from build123d import *

# Parameters (mm, degrees)
SKETCH_1_R          = 3.5
SKETCH_1_R_2        = 19
EXTRUDE_1_DEPTH     = 11.5
SKETCH_2_R          = 42.113859259
CUT_EXTRUDE_1_DEPTH = 6
SKETCH_3_R          = 15.5
CUT_EXTRUDE_3_DEPTH = 1
CUT_EXTRUDE_4_DEPTH = 1
FILLET_1_R          = 5
SKETCH_5_R          = 13.5
CUT_EXTRUDE_6_DEPTH = 21


with BuildPart() as part:
    # Эскиз1 → Бобышка-Вытянуть1 (new body)
    # profile 1 of 3: a face of its own
    with BuildSketch(Plane(origin=(0, 0, 0), x_dir=(1, 0, 0), z_dir=(0, 1, 0))):
        with BuildLine():
            ThreePointArc((-29.93902439, 6.351219512), (-31.061737619, 5.649390095), (-31.5, 4.4))
            Line((-31.5, 4.4), (-31.5, -4.4))
            ThreePointArc((-31.5, -4.4), (-31.061737619, -5.649390095), (-29.93902439, -6.351219512))
            Line((-29.93902439, -6.351219512), (-16.529826375, -9.368289066))
            ThreePointArc((-16.529826375, -9.368289066), (-19, 0), (-16.529826375, 9.368289066))
            Line((-16.529826375, 9.368289066), (-29.93902439, 6.351219512))
        make_face()
        with Locations(Location((-24, 0, 0), (0, 0, 270))):
            Circle(SKETCH_1_R, mode=Mode.SUBTRACT)
    # profile 2 of 3: a face of its own
    with BuildSketch(Plane(origin=(0, 0, 0), x_dir=(1, 0, 0), z_dir=(0, 1, 0))):
        Circle(SKETCH_1_R_2)
    # profile 3 of 3: a face of its own
    with BuildSketch(Plane(origin=(0, 0, 0), x_dir=(1, 0, 0), z_dir=(0, 1, 0))):
        with BuildLine():
            Line((29.93902439, 6.351219512), (16.529826375, 9.368289066))
            ThreePointArc((16.529826375, 9.368289066), (18.372080736, 4.844238788), (19, 0))
            ThreePointArc((19, 0), (18.372080736, -4.844238788), (16.529826375, -9.368289066))
            Line((16.529826375, -9.368289066), (29.93902439, -6.351219512))
            ThreePointArc((29.93902439, -6.351219512), (31.061737619, -5.649390095), (31.5, -4.4))
            Line((31.5, -4.4), (31.5, 4.4))
            ThreePointArc((31.5, 4.4), (31.061737619, 5.649390095), (29.93902439, 6.351219512))
        make_face()
        with Locations(Location((24, 0, 0), (0, 0, 270))):
            Circle(SKETCH_1_R, mode=Mode.SUBTRACT)
    extrude(amount=EXTRUDE_1_DEPTH)

    # Эскиз2 → Вырез-Вытянуть1 (cut)
    with BuildSketch(Plane(origin=(0, 11.5, 0), x_dir=(1, 0, 0), z_dir=(0, 1, 0))):
        Circle(SKETCH_2_R)
        with BuildLine():
            ThreePointArc((17.208333333, 3.1817077), (0, 17.5), (-17.208333333, 3.1817077))
            ThreePointArc((-17.208333333, 3.1817077), (-16.5, 0), (-17.208333333, -3.1817077))
            ThreePointArc((-17.208333333, -3.1817077), (0, -17.5), (17.208333333, -3.1817077))
            ThreePointArc((17.208333333, -3.1817077), (16.5, 0), (17.208333333, 3.1817077))
        make_face(mode=Mode.SUBTRACT)
    extrude(amount=-CUT_EXTRUDE_1_DEPTH, mode=Mode.SUBTRACT)

    # Эскиз3 → Вырез-Вытянуть3 (cut)
    with BuildSketch(Plane(origin=(0, 11.5, 0), x_dir=(1, 0, 0), z_dir=(0, 1, 0))):
        with Locations(Location((0, 0, 0), (0, 0, 270))):
            Circle(SKETCH_3_R)
    extrude(amount=-CUT_EXTRUDE_3_DEPTH, mode=Mode.SUBTRACT)

    # Эскиз4 → Вырез-Вытянуть4 (cut)
    with BuildSketch(Plane.XZ):
        with BuildLine():
            Line((-20.848643232, -5.321555273), (-15.718229563, -6.475898348))
            ThreePointArc((-15.718229563, -6.475898348), (-14.636214456, -8.647613914), (-13.256050789, -10.643172341))
            ThreePointArc((-13.256050789, -10.643172341), (-12.584964511, -11.011180012), (-11.850214134, -10.796871074))
            ThreePointArc((-11.850214134, -10.796871074), (-10.750830182, -10.362248437), (-9.598076211, -10.624355653))
            Line((-9.598076211, -10.624355653), (-4.401923789, -13.624355653))
            ThreePointArc((-4.401923789, -13.624355653), (-3.598555295, -14.491616268), (-3.425257564, -15.661022017))
            ThreePointArc((-3.425257564, -15.661022017), (-3.243479361, -16.404488978), (-2.58923223, -16.801662908))
            ThreePointArc((-2.58923223, -16.801662908), (8.351526577, -14.807160559), (15.718229563, -6.475898348))
            Line((15.718229563, -6.475898348), (20.848643232, -5.321555273))
            ThreePointArc((20.848643232, -5.321555273), (21.605203579, -4.563390663), (21.242016303, -3.555773605))
            ThreePointArc((21.242016303, -3.555773605), (19.5, 0), (21.242016303, 3.555773605))
            ThreePointArc((21.242016303, 3.555773605), (21.605203579, 4.563390663), (20.848643232, 5.321555273))
            Line((20.848643232, 5.321555273), (15.718229563, 6.475898348))
            ThreePointArc((15.718229563, 6.475898348), (14.636214456, 8.647613914), (13.256050789, 10.643172341))
            ThreePointArc((13.256050789, 10.643172341), (12.584964511, 11.011180012), (11.850214134, 10.796871074))
            ThreePointArc((11.850214134, 10.796871074), (10.750830182, 10.362248437), (9.598076211, 10.624355653))
            Line((9.598076211, 10.624355653), (4.401923789, 13.624355653))
            ThreePointArc((4.401923789, 13.624355653), (3.598555295, 14.491616268), (3.425257564, 15.661022017))
            ThreePointArc((3.425257564, 15.661022017), (3.243479361, 16.404488978), (2.58923223, 16.801662908))
            ThreePointArc((2.58923223, 16.801662908), (-8.351526577, 14.807160559), (-15.718229563, 6.475898348))
            Line((-15.718229563, 6.475898348), (-20.848643232, 5.321555273))
            ThreePointArc((-20.848643232, 5.321555273), (-21.605203579, 4.563390663), (-21.242016303, 3.555773605))
            ThreePointArc((-21.242016303, 3.555773605), (-19.5, 0), (-21.242016303, -3.555773605))
            ThreePointArc((-21.242016303, -3.555773605), (-21.605203579, -4.563390663), (-20.848643232, -5.321555273))
        make_face()
        with BuildLine():
            Line((6.035898385, 18.454482672), (12.964101615, 14.454482672))
            Line((12.964101615, 14.454482672), (11.464101615, 11.856406461))
            ThreePointArc((11.464101615, 11.856406461), (10.856895256, 11.390480634), (10.098076211, 11.490381057))
            Line((10.098076211, 11.490381057), (4.901923789, 14.490381057))
            ThreePointArc((4.901923789, 14.490381057), (4.435997962, 15.097587415), (4.535898385, 15.856406461))
            Line((4.535898385, 15.856406461), (6.035898385, 18.454482672))
        make_face()
        with BuildLine():
            Line((-6.035898385, -18.454482672), (-4.535898385, -15.856406461))
            ThreePointArc((-4.535898385, -15.856406461), (-4.435997962, -15.097587415), (-4.901923789, -14.490381057))
            Line((-4.901923789, -14.490381057), (-10.098076211, -11.490381057))
            ThreePointArc((-10.098076211, -11.490381057), (-10.856895256, -11.390480634), (-11.464101615, -11.856406461))
            Line((-11.464101615, -11.856406461), (-12.964101615, -14.454482672))
            Line((-12.964101615, -14.454482672), (-6.035898385, -18.454482672))
        make_face()
    extrude(amount=-CUT_EXTRUDE_4_DEPTH, mode=Mode.SUBTRACT)

    # Скругление1
    fillet_1_edges = [part.edges().sort_by_distance(p)[0] for p in [
        (-16.529826375, 2.75, -9.368289066),
        (16.529826375, 2.75, -9.368289066),
        (16.529826375, 2.75, 9.368289066),
        (-16.529826375, 2.75, 9.368289066),
    ]]
    fillet(fillet_1_edges, radius=FILLET_1_R)

    # Эскиз5 → Вырез-Вытянуть6 (cut)
    with BuildSketch(Plane(origin=(0, 10.5, 0), x_dir=(1, 0, 0), z_dir=(0, 1, 0))):
        with Locations(Location((0, 0, 0), (0, 0, 270))):
            Circle(SKETCH_5_R)
    extrude(amount=-CUT_EXTRUDE_6_DEPTH, mode=Mode.SUBTRACT)


solid = part.part
Work out the finished part from the listing and answer in its coordinate system (mm). A direction names the side the tool comes from. Round coordinates to 2 decimals unless told otherwise and drop trailing zeros. Write each loop counter-clockwise with the first axis right and the second up, starting at its lowest first coordinate (ties: lowest second). Pieces come first, ordered by that corner, then holes.
1) Given pin 1 Ø3 at (y, z) = (7.5, 13.5) entering from +X; pin 2 Ø6 at (y, z) = (10, -12) entering from +X; pin 3 Ø5 at (x, z) = (17.5, 13) entering from +Y; pin 4 Ø5.5 at (x, z) = (8, 16) entering from -Y, each flat-ended and moving along its own axis, determine where each tip first touches the part or whether it passes through.
2) A cutting plane is placed at C-C (z = 12.5). Give the vertices of the cut face in (x, y).
3) A cutting plane is placed at D-D (x = -25). Give the vertices of the cut face in (y, z), plus the area to 3 significant figures.
4) A cutting plane is placed at A-A (x = 0). Give the vertices of the cut face in (y, z).
5) Straight lines are drawn through the part: line 1 (X direction, y = 3.3, z = 0); line 2 (X direction, y = 1.25, z = -1); line 3 (X direction, y = 6.5, z = 0). For each, find the intervals that lie inside material, in ascending order.
6) The mould has two halves that part along Z. Classify faces 5 (the cylindrical face through (-19.5, 0.5, 0.1)), 6 (the cylindrical face through (0.34, 8.542, -17.497)), 7 (the flat face through (-24.321, 2.712, 7.615)): pulls with the +Z half, pulls with the -Z half, needs draft (parallel to the pull), parting line crosses it, or undercut.
7) A tool of negligible diameter and unlimited length cuts with its end or side. For faces 1 (the flat face through (-18.248, 0.493, 5.907)), 2 (the flat face through (13, 10.5, -5)), 3 (the flat face through (5.17, 0.493, 16.955)), 4 (the cylindrical face through (-16.5, 8.5, 0)), from which of +Z, -Z, +X, -X, +Y, -Y can it reach the whole face along a straight path? Write none if from no direction.
8) A cutting plane is placed at B-B (y = 2.5). Give the vertices of the cut face in (x, z), plus the area to 3 significant figures.
Completed:
1. pin 1: stops at x = 12.74
1. pin 2: stops at x = 15.01
1. pin 3: passes through
1. pin 4: stops at y = 1
2. outline: (-14.31, 0) - (-11.52, 0) - (-11.52, 1) - (-5.1, 1) - (-5.1, 10.5) - (-9.17, 10.5) - (-9.17, 11.5) - (-12.25, 11.5) - (-12.25, 5.5) - (-14.31, 5.5) - close; (5.1, 1) - (6.35, 1) - (6.35, 0) - (8.35, 0) - (8.35, 1) - (11.84, 1) - (11.84, 0) - (14.31, 0) - (14.31, 5.5) - (12.25, 5.5) - (12.25, 11.5) - (9.17, 11.5) - (9.17, 10.5) - (5.1, 10.5) - close
3. outline: (0, -7.46) - (5.5, -7.46) - (5.5, -3.35) - (0, -3.35) - close; (0, 3.35) - (5.5, 3.35) - (5.5, 7.46) - (0, 7.46) - close
3. area: 45.2 mm2
4. outline: (0, -19) - (5.5, -19) - (5.5, -17.5) - (11.5, -17.5) - (11.5, -15.5) - (10.5, -15.5) - (10.5, -13.5) - (1, -13.5) - (1, -17) - (0, -17) - close; (0, 17) - (1, 17) - (1, 13.5) - (10.5, 13.5) - (10.5, 15.5) - (11.5, 15.5) - (11.5, 17.5) - (5.5, 17.5) - (5.5, 19) - (0, 19) - close
5. line 1: x = -31.5 to -27.5, -20.5 to -13.5, 13.5 to 20.5, 27.5 to 31.5
5. line 2: x = -31.5 to -27.35, -20.65 to -13.46, 13.46 to 20.65, 27.35 to 31.5
5. line 3: x = -16.5 to -13.5, 13.5 to 16.5
6. face 5: undercut
6. face 6: pulls with the -Z half
6. face 7: pulls with the +Z half
7. face 1: -Y
7. face 2: +Y
7. face 3: +X, -Y
7. face 4: -X, +Y
8. outline: (-31.5, -4.4) arc R2 ccw to (-29.94, -6.35) - (-18.54, -8.92) arc R5 cw to (-15.55, -10.92) arc R19 ccw to (15.55, -10.92) arc R5 cw to (18.54, -8.92) - (29.94, -6.35) arc R2 ccw to (31.5, -4.4) - (31.5, 4.4) arc R2 ccw to (29.94, 6.35) - (18.54, 8.92) arc R5 cw to (15.55, 10.92) arc R19 ccw to (-15.55, 10.92) arc R5 cw to (-18.54, 8.92) - (-29.94, 6.35) arc R2 ccw to (-31.5, 4.4) - close; hole circle Ø7 at (-24, 0); hole circle Ø27 at (0, 0); hole circle Ø7 at (24, 0)
8. area: 882 mm2
